The listing builds one solid part. Answer for the finished solid, in the listing's coordinates (mm). A direction names the side the tool comes from. Coordinates: 2 decimals unless noted, no trailing zeros. Write each loop counter-clockwise with the first axis right and the second up, starting at its lowest first coordinate (ties: lowest second). Pieces come first, ordered by that corner, then holes.
(1) Given P1, Ø4, axis at x = 7, y = 2, coming from the +Z side; P2, Ø0.8, axis at x = 26.5, z = 5.5, coming from the +Y side (3 decimals), each flat-ended and moving along its own axis, determine where each tip first touches the part or whether it passes through.
(2) Straight lines are drawn through the part: line 1 (X direction, y = -9, z = 4); line 2 (Y direction, x = 16.5, z = 7.25); line 3 (X direction, y = 9.5, z = 1). For each, find the intervals that lie inside material, in ascending order.
(3) The part is cut by section D-D on z = 5.25. Determine the outline of the cut face in (x, y), plus the area to 3 significant figures.
(4) For a pull along Y with two mould halves and no side action, classify faces 1 (the flat face through (0, 17, 9)), 2 (the cylindrical face through (26.493, -4.699, 7.715)), 3 (the cylindrical face through (26.699, -16.715, 9.633)) as +Y half, -Y half, draft (parallel to the pull), parting line (faces both ways), or undercut.
(5) Which of the six approach directions +Z, -Z, +X, -X, +Y, -Y give full straight-line access (tool end or side, diameter ignored) to faces 4 (the flat face through (11, 0, 2)), 5 (the cylindrical face through (26.699, 16.715, 9.367)), 6 (the cylindrical face through (26.493, -4.699, 3.285)), 7 (the flat face through (0, -17, 9)), 8 (the flat face through (-10, -14, 1))?
(6) The part is cut by section A-A on x = -22. Determine the outline of the cut face in (y, z), plus the area to 3 significant figures.
(7) The part is cut by section C-C on z = 11.75. Determine the outline of the cut face in (x, y), plus the area to 3 significant figures.
(8) The part is cut by section B-B on y = -11. Determine the outline of the cut face in (x, z).
from build123d import *

# Parameters (mm, degrees)
SKETCH1_W           = 54
SKETCH1_H           = 34
SKETCH1_W_2         = 28
SKETCH1_H_2         = 28
BOSS_EXTRUDE1_DEPTH = 2
SKETCH2_W           = 54
SKETCH2_H           = 34
SKETCH2_W_2         = 52
SKETCH2_H_2         = 32
BOSS_EXTRUDE2_DEPTH = 17
FILLET1_R           = 1
FILLET2_R           = 1
SKETCH3_W           = 5
SKETCH3_H           = 10
CUT_EXTRUDE1_DEPTH  = 17
FILLET3_R           = 1
FILLET4_R           = 1


with BuildPart() as part:
    # Sketch1 → Boss-Extrude1 (new body)
    with BuildSketch(Plane.XY):
        Rectangle(SKETCH1_W, SKETCH1_H)
        with Locations((-10, 0)):
            Rectangle(SKETCH1_W_2, SKETCH1_H_2, mode=Mode.SUBTRACT)
    extrude(amount=BOSS_EXTRUDE1_DEPTH)

    # Sketch2 → Boss-Extrude2 (add)
    with BuildSketch(Plane.XY.offset(2)):
        Rectangle(SKETCH2_W, SKETCH2_H)
        Rectangle(SKETCH2_W_2, SKETCH2_H_2, mode=Mode.SUBTRACT)
    extrude(amount=BOSS_EXTRUDE2_DEPTH)

    # Fillet1
    fillet1_edges = [part.edges().sort_by_distance(p)[0] for p in [
        (26, 16, 10.5),
        (-26, 16, 10.5),
        (-26, -16, 10.5),
        (26, -16, 10.5),
    ]]
    fillet(fillet1_edges, radius=FILLET1_R)

    # Fillet2
    fillet2_edges = [part.edges().sort_by_distance(p)[0] for p in [
        (27, -17, 9.5),
        (-27, -17, 9.5),
        (-27, 17, 9.5),
        (27, 17, 9.5),
    ]]
    fillet(fillet2_edges, radius=FILLET2_R)

    # Sketch3 → Cut-Extrude1 (cut)
    with BuildSketch(Plane(origin=(27, 0, 0), x_dir=(0, 0, -1), z_dir=(1, 0, 0))):
        with Locations((-5.5, 0)):
            Rectangle(SKETCH3_W, SKETCH3_H)
    extrude(amount=-CUT_EXTRUDE1_DEPTH, mode=Mode.SUBTRACT)

    # Fillet3
    fillet3_edges = [part.edges().sort_by_distance(p)[0] for p in [
        (26.5, 5, 3),
        (26.5, -5, 3),
        (26.5, -5, 8),
        (26.5, 5, 8),
    ]]
    fillet(fillet3_edges, radius=FILLET3_R)

    # Fillet4
    fillet4_edges = [part.edges().sort_by_distance(p)[0] for p in [
        (4, -14, 1),
        (4, 14, 1),
        (-24, 14, 1),
        (-24, -14, 1),
    ]]
    fillet(fillet4_edges, radius=FILLET4_R)


solid = part.part
Model answer:
1. P1: stops at z = 2
1. P2: stops at y = 16.995
2. line 1: x = -27 to -26, 26 to 27
2. line 2: y = -17 to -16, 16 to 17
2. line 3: x = -27 to -24, 4 to 27
3. outline: (-27, -16) arc R1 ccw to (-26, -17) - (26, -17) arc R1 ccw to (27, -16) - (27, -5) - (26, -5) - (26, -15) arc R1 cw to (25, -16) - (-25, -16) arc R1 cw to (-26, -15) - (-26, 15) arc R1 cw to (-25, 16) - (25, 16) arc R1 cw to (26, 15) - (26, 5) - (27, 5) - (27, 16) arc R1 ccw to (26, 17) - (-26, 17) arc R1 ccw to (-27, 16) - close
3. area: 162 mm2
4. face 1: +Y half
4. face 2: undercut
4. face 3: -Y half
5. face 4: +Z
5. face 5: +Z, -Z, +X, +Y
5. face 6: +X
5. face 7: +Z, -Z, +X, -X, -Y
5. face 8: +Z, -Z
6. outline: (-17, 0) - (-14, 0) - (-14, 2) - (-16, 2) - (-16, 19) - (-17, 19) - close; (14, 0) - (17, 0) - (17, 19) - (16, 19) - (16, 2) - (14, 2) - close
6. area: 46.0 mm2
7. outline: (-27, -16) arc R1 ccw to (-26, -17) - (26, -17) arc R1 ccw to (27, -16) - (27, 16) arc R1 ccw to (26, 17) - (-26, 17) arc R1 ccw to (-27, 16) - close; hole (-26, -15) arc R1 ccw to (-25, -16) - (25, -16) arc R1 ccw to (26, -15) - (26, 15) arc R1 ccw to (25, 16) - (-25, 16) arc R1 ccw to (-26, 15) - close
7. area: 172 mm2
8. outline: (-27, 0) - (-24, 0) - (-24, 2) - (-26, 2) - (-26, 19) - (-27, 19) - close; (4, 0) - (27, 0) - (27, 19) - (26, 19) - (26, 2) - (4, 2) - close
